Build history of the part. All positions in model axes, mm. Give positions to 0.01 mm unless a question says otherwise; leave off trailing zeros. Write each loop counter-clockwise with the first axis right and the second up, starting at its lowest first coordinate (ties: lowest second). Pieces come first, ordered by that corner, then holes. Notation, with made-up numbers: M 31.25,-14.75 L 80.25,-14.75 A17 cw 80.25,-5.75 Z; hole C 5.5,50.5 d1. An arc over 180 degrees is marked long. Return JSON: item names as keys, results as strings. Group by question number.
Q1. Band-saw the part on D-D, the plane z = -30. Give the cut face in (x, y), then the cut area to 3 significant figures.
Q2. Flat gauge pins, fed straight in: pin 1 Ø2.5 at (x, z) = (10, -67.5) entering from +Y; pin 2 Ø1.5 at (y, z) = (1, -49.5) entering from -X. Where does each tip first touch, or does it go through?
Q3. Band-saw the part on C-C, the plane z = 67.5. Give the cut face in (x, y), then the cut area to 3 significant figures.
Q4. Band-saw the part on A-A, the plane y = 0.5. Give the cut face in (x, z), then the cut area to 3 significant figures.
Q5. Band-saw the part on B-B, the plane x = -10. Give the cut face in (y, z).
Q6. Wall check: probe 1 along X at (y, z) = (2.1, 67.5); probe 2 along X at (y, z) = (1.2, -67.5); probe 3 along Z at (x, y) = (-11, 1). Give the ranges that are in metal, low to high.
from build123d import *

# Parameters (mm, degrees)
SKETCH1_W           = 50
SKETCH1_H           = 140
BOSS_EXTRUDE2_DEPTH = 5
CUT_EXTRUDE1_DEPTH  = 152
SKETCH7_W           = 50
SKETCH7_H           = 2
CUT_EXTRUDE5_DEPTH  = 197
SKETCH8_W           = 30
SKETCH8_H           = 130
CUT_EXTRUDE6_DEPTH  = 197
SKETCH9_W           = 40
SKETCH9_H           = 20
SKETCH9_R           = 1.5
BOSS_EXTRUDE5_DEPTH = 3
SKETCH10_W          = 30
SKETCH10_H          = 10
SKETCH10_R          = 1.5
BOSS_EXTRUDE6_DEPTH = 3
SKETCH11_R          = 1.5
CUT_EXTRUDE7_DEPTH  = 3
SKETCH12_W          = 30.040139405
SKETCH12_H          = 126.520437971
BOSS_EXTRUDE8_DEPTH = 3


with BuildPart() as part:
    # Sketch1 → Boss-Extrude2 (new body)
    with BuildSketch(Plane(origin=(0, 0, 0), x_dir=(1, 0, 0), z_dir=(0, 1, 0))):
        Rectangle(SKETCH1_W, SKETCH1_H)
    extrude(amount=BOSS_EXTRUDE2_DEPTH)

    # Sketch2 → Cut-Extrude1 (cut)
    with BuildSketch(Plane.XY.offset(70)):
        Polygon((-20, 0), (-25, 5), (-25, 0), align=None)
        Polygon((25, 5), (20, 0), (25, 0), align=None)
    extrude(amount=-CUT_EXTRUDE1_DEPTH, mode=Mode.SUBTRACT)

    # Sketch7 → Cut-Extrude5 (cut)
    with BuildSketch(Plane(origin=(0, 0, -70), x_dir=(-1, 0, 0), z_dir=(0, 0, -1))):
        with Locations((0, 4)):
            Rectangle(SKETCH7_W, SKETCH7_H)
    extrude(amount=-CUT_EXTRUDE5_DEPTH, mode=Mode.SUBTRACT)

    # Sketch8 → Cut-Extrude6 (cut)
    with BuildSketch(Plane.XZ):
        Rectangle(SKETCH8_W, SKETCH8_H)
    extrude(amount=-CUT_EXTRUDE6_DEPTH, mode=Mode.SUBTRACT)

    # Sketch9 → Boss-Extrude5 (add)
    with BuildSketch(Plane.XZ):
        with Locations((0, -60)):
            Rectangle(SKETCH9_W, SKETCH9_H)
        with Locations(Location((-13.5, -56.5, 0), (0, 0, 270))):
            Circle(SKETCH9_R, mode=Mode.SUBTRACT)
        with Locations(Location((13.5, -56.5, 0), (0, 0, 90))):
            Circle(SKETCH9_R, mode=Mode.SUBTRACT)
    extrude(amount=-BOSS_EXTRUDE5_DEPTH)

    # Sketch10 → Boss-Extrude6 (add)
    with BuildSketch(Plane.XZ):
        with Locations((0, 50)):
            Rectangle(SKETCH10_W, SKETCH10_H)
        with Locations(Location((-10, 50, 0), (0, 0, 270))):
            Circle(SKETCH10_R, mode=Mode.SUBTRACT)
        with Locations(Location((10, 50, 0), (0, 0, 270))):
            Circle(SKETCH10_R, mode=Mode.SUBTRACT)
    extrude(amount=-BOSS_EXTRUDE6_DEPTH)

    # Sketch11 → Cut-Extrude7 (cut)
    with BuildSketch(Plane.XZ):
        with Locations(Location((-10, 67.5, 0), (0, 0, 270))):
            Circle(SKETCH11_R)
        with Locations(Location((10, 67.5, 0), (0, 0, 90))):
            Circle(SKETCH11_R)
        with Locations(Location((10, -67.5, 0), (0, 0, 270))):
            Circle(SKETCH11_R)
        with Locations(Location((-10, -67.5, 0), (0, 0, 90))):
            Circle(SKETCH11_R)
    extrude(amount=-CUT_EXTRUDE7_DEPTH, mode=Mode.SUBTRACT)

    # Sketch12 → Boss-Extrude8 (add)
    with BuildSketch(Plane(origin=(0, 3, 0), x_dir=(1, 0, 0), z_dir=(0, 1, 0))):
        with Locations((-0.020069702, -1.739781014)):
            Rectangle(SKETCH12_W, SKETCH12_H)
    extrude(amount=-BOSS_EXTRUDE8_DEPTH)


solid = part.part
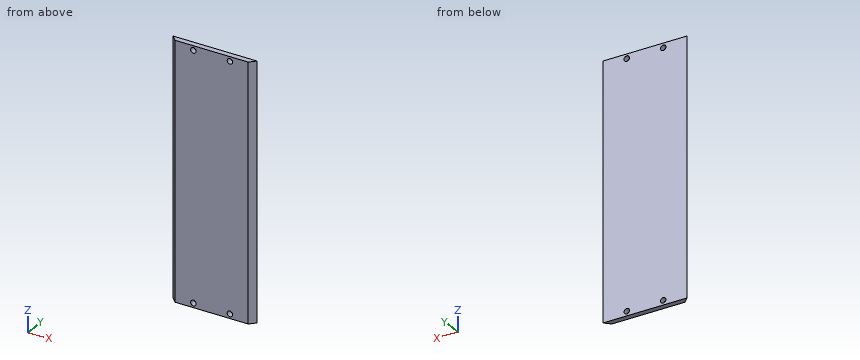
From the geometry:
{
 "1": {"outline": "M -23,3 L -20,0 L 20,0 L 23,3 Z", "area": "129 mm^2"},
 "2": {"pin 1": "passes through", "pin 2": "stops at x = -21.75"},
 "3": {"outline": "M -23,3 L -20,0 L -11.5,0 L -11.5,3 Z; M -8.5,0 L 8.5,0 L 8.5,3 L -8.5,3 Z; M 11.5,0 L 20,0 L 23,3 L 11.5,3 Z", "area": "111 mm^2"},
 "4": {"outline": "M -20.5,-70 L 20.5,-70 L 20.5,70 L -20.5,70 Z; hole C -10,-67.5 d3; hole C -10,67.5 d3; hole C 10,-67.5 d3; hole C 10,67.5 d3", "area": "5,710 mm^2"},
 "5": {"outline": "M 0,-70 L 3,-70 L 3,-69 L 0,-69 Z; M 0,-66 L 3,-66 L 3,66 L 0,66 Z; M 0,69 L 3,69 L 3,70 L 0,70 Z"},
 "6": {"probe 1": "x = -22.1 to -11.5, -8.5 to 8.5, 11.5 to 22.1", "probe 2": "x = -21.2 to -11.5, -8.5 to 8.5, 11.5 to 21.2", "probe 3": "z = -70 to -68.62, -66.38 to 66.38, 68.62 to 70"}
}
